Source: CAD feature listing. Evaluate the final solid. Frame: model axes, mm. A direction names the side the tool comes from. Round coordinates to 2 decimals unless told otherwise and drop trailing zeros. Order: outer loops, then holes, each group sorted by start corner. A loop starts at its lowest first (then second) coordinate and runs counter-clockwise, first axis right, second up. Notation, with made-up numbers: (79, 34.5) -> (133, 34.5) arc R10 ccw to (133, 41.5) -> close; hole circle Ø1 at (67, 51). An arc over 180 degrees is marked (long way). One line per item, written item: value. Start each with the question number.
1) Section B-B (x = 0). Return the cut outline in (y, z), and give its area (3 significant figures).
2) Pin query (flat end, axial travel): P1, Ø5, axis at y = 11, z = -3, coming from the +X side; P2, Ø1.5, axis at y = 23, z = 7.5, coming from the +X side; P3, Ø7, axis at x = 0, z = 0, coming from the +Y side. Return the tip coordinate at first contact, or that it passes through.
3) Reachability of faces 1 (the face through (7.325, 6.11, -3.81)), 2 (the face through (5.37, 43.55, 1.19)) from +Z, -Z, +X, -X, +Y, -Y: full face, straight path, thin tool, end or side. Return the list, or none.
4) Ray query, L1, parallel to X at y = 23, z = 0; L2, parallel to Z at x = 6, y = 40; L3, parallel to Z at x = -1.5, y = 28. Return the intervals inside material, ascending.
5) Section D-D (y = 17.5). Return the cut outline in (x, z).
6) Section A-A (z = 0). Return the cut outline in (x, y).
7) Section C-C (y = 41). Return the cut outline in (x, z), and give its area (3 significant figures).
8) Mould query, pull axis Z, two halves, no side actions, for faces 3 (the face through (0, 30, 10)), 4 (the face through (-5.4, 47, 1.7)), 5 (the face through (2.4, 40, 2.4)). Classes: pulls with the +Z half, pulls with the -Z half, needs draft (parallel to the pull), parting line crosses it, or undercut.
```python
from build123d import *

# Parameters (mm, degrees)
CONG_1_R = 2


with BuildPart() as part:
    # Esquisse1 → Révolution1 (revolve)
    with BuildSketch(Plane.XY, mode=Mode.PRIVATE) as r_volution1_sk:
        Polygon((3.1, 0), (3.1, 40), (5.5, 40), (5.5, 47), (10, 47), (10, 16), (7.178768309, 0), align=None)
    revolve(r_volution1_sk.sketch.rotate(Axis((0, 0, 0), (0, 1, 0)), 90), axis=Axis((0, 0, 0), (0, 1, 0)))

    # Congé1
    cong_1_edges = [part.edges().sort_by_distance(p)[0] for p in [
        (0, 47, 10),
    ]]
    fillet(cong_1_edges, radius=CONG_1_R)


solid = part.part
```
Findings:
1. outline: (0, -7.18) -> (16, -10) -> (45, -10) arc R2 ccw to (47, -8) -> (47, -5.5) -> (40, -5.5) -> (40, -3.1) -> (0, -3.1) -> close; (0, 3.1) -> (40, 3.1) -> (40, 5.5) -> (47, 5.5) -> (47, 8) arc R2 ccw to (45, 10) -> (16, 10) -> (0, 7.18) -> close
1. area: 568 mm2
2. P1: x = 9.35
2. P2: x = 7.38
2. P3: y = 40
3. face 1: -Y
3. face 2: +Y
4. L1: -10 to -3.1, 3.1 to 10
4. L2: -8 to 8
4. L3: -9.89 to -2.71, 2.71 to 9.89
5. outline: circle Ø20 at (0, 0); hole circle Ø6.2 at (0, 0)
6. outline: (-10, 16) -> (-7.18, 0) -> (-3.1, 0) -> (-3.1, 40) -> (-5.5, 40) -> (-5.5, 47) -> (-8, 47) arc R2 ccw to (-10, 45) -> close; (3.1, 0) -> (7.18, 0) -> (10, 16) -> (10, 45) arc R2 ccw to (8, 47) -> (5.5, 47) -> (5.5, 40) -> (3.1, 40) -> close
7. outline: circle Ø20 at (0, 0); hole circle Ø11 at (0, 0)
7. area: 219 mm2
8. face 3: parting line crosses it
8. face 4: needs draft
8. face 5: undercut
